Part model, mm, in its own coordinate system. A direction names the side the tool comes from. Round coordinates to 2 decimals unless told otherwise and drop trailing zeros. Loops run counter-clockwise (first coordinate to the right, second up) from the corner with the lowest first, then second, coordinate; pieces in that order, holes last.
(1) Mould opens along Z. For faces 4 (the face through (0, 0, 12.7)), 5 (the face through (-18, -12.785, 0)), 6 (the face through (1, 21.505, 11)) say: +Z half, -Z half, draft (parallel to the pull), parting line (faces both ways), or undercut.
(2) Tool access for faces 1 (the face through (23, -8.975, 41)), 2 (the face through (20, 0, -6.35)), 3 (the face through (-9.57, 5.85, 9.57)): list every direction of +Z, -Z, +X, -X, +Y, -Y with a clear straight run to the whole face (end or side of a thin tool).
(3) Flat gauge pins, fed straight in: pin 1 (5 mm diameter, centred on x = 8.5, y = 8, fed in from +Z); pin 2 (4 mm diameter, centred on x = 15.5, y = -12, fed in from -Z); pin 3 (8 mm diameter, centred on x = 6.5, z = -12.5, fed in from +Y); pin 4 (5 mm diameter, centred on x = 22, y = -1.5, fed in from +Z). Where does each tip first touch, or does it go through?
(4) Probe probe 1 along Y at (x, z) = (12.7, 10.25); probe 2 along X at (y, z) = (-11, -7) (3 decimals); probe 3 along X at (y, z) = (12, 33) (3 decimals). List the from-to ranges inside material, lowest first.
(5) Cut at B-B on z = 31.5. List the corners of the cut face in (x, y) (3 decimals), then the cut area to 3 significant figures.
(6) Cut at C-C on x = -16. List the corners of the cut face in (y, z).
Autodesk Inventor part; units mm, degrees
ref_plane "YZ Plane" through (0, 0, 0) normal (1, 0, 0) x (0, 1, 0)
ref_plane "XZ Plane" through (0, 0, 0) normal (0, 1, 0) x (-1, 0, 0)
ref_plane "XY Plane" through (0, 0, 0) normal (0, 0, 1) x (1, 0, 0)
sketch "Sketch1" plane through (0, 0, 0) normal (0, 0, 1) x (1, 0, 0)
  line L0 (-15.24, 10.0753) -> (16.51, 10.0753)
  line L1 (16.51, 10.0753) -> (16.51, -15.3247)
  line L2 (16.51, -15.3247) -> (-15.24, -15.3247)
  line L3 (-15.24, -15.3247) -> (-15.24, 10.0753)
  circle A0 centre (-11.43, 6.2653) radius 1.905
  circle A1 centre (-11.43, -6.4347) radius 1.905
  circle A2 centre (12.7, 6.2653) radius 1.905
  circle A3 centre (12.7, -6.4347) radius 1.905
  point P0 (0, 0)
  dimension "d0" = 31.75
  dimension "d1" = 25.4
  dimension "d10" = 3.81
  dimension "d11" = 8.89
  dimension "d12" = 3.81
  dimension "d13" = 3.81
  dimension "d14" = 8.89
  dimension "d15" = 3.81
  dimension "d16" = 3.81
  dimension "d17" = 3.81
  dimension "d18" = 3.81
  dimension "d19" = 3.81
  dimension "d20" = 3.81
  dimension "d21" = 3.81
  dimension "d22" = 8.89
extrude "Extrusion1" add sketch "Sketch1" along normal blind 6.35
sketch "Sketch2" plane through (0, 0, 6.35) normal (0, 0, 1) x (1, 0, 0)
  line L0 (-24.765, 16.4253) -> (26.035, 16.4253)
  line L1 (26.035, 16.4253) -> (26.035, -21.6747)
  line L2 (26.035, -21.6747) -> (-24.765, -21.6747)
  line L3 (-24.765, -21.6747) -> (-24.765, 16.4253)
  line L4 (16.51, -15.3247) -> (16.51, 10.0753)
  line L5 (-15.24, 10.0753) -> (-15.24, -15.3247)
  line L6 (16.51, 10.0753) -> (-15.24, 10.0753)
  point P0 (0, 0)
  dimension "d25" = 50.8
  dimension "d26" = 38.1
  dimension "d27" = 9.525
  dimension "d29" = 9.525
  dimension "d30" = 6.35
extrude "Extrusion2" add sketch "Sketch2" along normal blind 6.35
sketch "Sketch3" plane through (0, 0, 6.35) normal (0, 0, -1) x (-1, 0, 0)
  line L0 (24.765, -21.6747) -> (24.765, 16.4253)
  circle A0 centre (11.43, 6.2653) radius 1.905
  line L1 (24.765, 16.4253) -> (-26.035, 16.4253)
  circle A1 centre (11.43, -6.4347) radius 1.905
  line L2 (-26.035, -21.6747) -> (24.765, -21.6747)
  line L3 (-26.035, 16.4253) -> (-26.035, -21.6747)
  point P0 (0, 0)
  point P1 (-12.7, -6.4347)
  point P2 (-12.7, 6.2653)
  dimension "d33" = 13.335
  dimension "d34" = 10.16
  dimension "d35" = 13.335
  dimension "d36" = 15.24
  dimension "d37" = 13.335
  dimension "d38" = 10.16
  dimension "d39" = 15.24
  dimension "d40" = 13.335
hole "Hole1" at (-11.43, 6.2653, 6.35) at (-11.43, -6.4347, 6.35) at (12.7, -6.4347, 6.35) at (12.7, 6.2653, 6.35) direction (0, 0, 1) diameter 3.81 end through all
sketch "Sketch4" plane through (0, 0, 12.7) normal (0, 0, 1) x (1, 0, 0)
  line L0 (26.035, 16.4253) -> (26.035, -21.6747)
  line L1 (26.035, 16.4253) -> (19.685, 16.4253)
  line L2 (19.685, 16.4253) -> (19.685, -21.6747)
  line L3 (19.685, -21.6747) -> (26.035, -21.6747)
  line L4 (26.035, -21.6747) -> (26.035, 16.4253)
  line L5 (-24.765, 16.4253) -> (26.035, 16.4253)
  line L6 (-24.765, 16.4253) -> (-18.415, 16.4253)
  line L7 (-18.415, 16.4253) -> (-18.415, -21.6747)
  line L8 (-18.415, -21.6747) -> (-24.765, -21.6747)
  line L9 (-24.765, -21.6747) -> (-24.765, 16.4253)
  point P0 (0, 0)
  dimension "d48" = 6.35
  dimension "d49" = 6.35
extrude "Extrusion3" add sketch "Sketch4" along normal blind 34.925
sketch "Sketch5" plane through (26.035, -21.6747, 6.35) normal (1, 0, 0) x (0, 0, -1)
  line L0 (-41.2903, 25.4) -> (-28.2305, 25.4)
  line L1 (-28.2305, 25.4) -> (-28.2305, 12.7)
  line L2 (-28.2305, 12.7) -> (-41.2903, 12.7)
  line L3 (-41.2903, 12.7) -> (-41.2903, 25.4)
  line L4 (0, 38.1) -> (-41.275, 38.1)
  point P0 (6.35, 21.6747)
  dimension "d52" = 12.7
  dimension "d53" = 12.7
extrude "Extrusion4" cut sketch "Sketch5" against normal through all
sketch "Sketch6" plane through (0, 0, 6.35) normal (0, 0, -1) x (-1, 0, 0)
  point P0 (0, 0)
sketch "Sketch7" plane through (0, 0, 6.35) normal (0, 0, -1) x (-1, 0, 0)
  line L0 (-26.035, 16.4253) -> (-26.035, -21.6747)
  line L1 (24.765, -21.6747) -> (18.415, -21.6747)
  line L2 (-26.035, 16.4253) -> (24.765, 16.4253)
  line L3 (24.765, 16.4253) -> (24.765, -21.6747)
  line L4 (24.765, -21.6747) -> (-26.035, -21.6747)
  line L5 (-26.035, -21.6747) -> (-26.035, 16.4253)
  point P0 (0, 0)
extrude "Extrusion5" add sketch "Sketch7" along normal blind 32.385
sketch "Sketch8" plane through (-18.415, -21.6747, 12.7) normal (0, -1, 0) x (1, 0, 0)
  line L0 (44.45, -38.735) -> (-6.35, -38.735)
  line L1 (44.45, 34.925) -> (44.45, -38.735)
  line L2 (0, 0) -> (38.1, 0)
  line L3 (-6.35, 34.925) -> (-6.35, -38.735)
  point P0 (18.415, -12.7)
  point P1 (19.05, -19.3675)
  dimension "d60" = 19.3675
  dimension "d61" = 25.4
  dimension "d62" = 19.3675
  dimension "d63" = 25.4
hole "Hole2" at (0.635, -21.6747, -6.6675) direction (0, 1, 0) diameter 26.797 end through all
fillet "Fillet3" radius 12.7 2 edges at (-24.765, -2.6247, -26.035) (26.035, -2.6247, -26.035)
sketch "Sketch9" plane through (0, 0, 12.7) normal (0, 0, 1) x (1, 0, 0)
  circle A0 centre (12.7, -6.4347) radius 1.905
  circle A1 centre (-11.43, -6.4347) radius 1.905
  circle A2 centre (-11.43, 6.2653) radius 1.905
  line L0 (-18.415, -21.6747) -> (19.685, -21.6747)
  line L1 (26.035, 3.7253) -> (26.035, -8.9747)
  circle A3 centre (12.7, 6.2653) radius 1.905
  circle A4 centre (-11.43, -6.4347) radius 1.905
  circle A5 centre (12.7, 6.2653) radius 1.905
  line L2 (19.685, 16.4253) -> (-18.415, 16.4253)
  point P0 (0, 0)
  dimension "d73" = 15.24
  dimension "d74" = 13.335
  dimension "d75" = 12.7
  dimension "d76" = 24.13
  dimension "d77" = 24.13
  dimension "d78" = 3.81
  dimension "d79" = 3.81
  dimension "d80" = 12.7
  dimension "d81" = 3.81
  dimension "d82" = 10.16
  dimension "d83" = 24.13
extrude "Extrusion6" cut sketch "Sketch9" against normal blind 19.05
sketch "Sketch10" plane through (26.035, 3.7253, 47.625) normal (1, 0, 0) x (0, 0, -1)
  line L0 (41.275, 8.89) -> (53.975, 8.89)
  line L1 (53.975, 8.89) -> (53.975, -16.51)
  line L2 (53.975, -16.51) -> (41.275, -16.51)
  line L3 (41.275, -16.51) -> (41.275, 8.89)
  line L4 (34.925, -25.4) -> (34.925, 12.7)
  line L5 (0, 12.7) -> (60.96, 12.7)
  point P0 (47.625, -3.7253)
  dimension "d86" = 12.7
  dimension "d87" = 25.4
  dimension "d88" = 6.35
  dimension "d91" = 3.81
extrude "Extrusion7" cut sketch "Sketch10" against normal through all
thicken "Thicken1" operation add thickness 5.08 both sides no extend neighbours yes toward (0, 1, 0) faces at (-22.6483, 16.4253, 15.6633)
sketch "Sketch11" plane through (-18.415, 21.5053, 12.7) normal (0, 1, 0) x (1, 0, 0)
  point P0 (18.415, 12.7)
sketch "Sketch12" plane through (-24.765, -21.6747, 47.625) normal (-1, 0, 0) x (0, 0, 1)
  line L0 (-60.96, 43.18) -> (0, 43.18)
  line L1 (0, 0) -> (-60.96, 0)
  point P0 (-47.625, 21.6747)
sketch "Sketch13" plane through (-18.415, 21.5053, 12.7) normal (0, 1, 0) x (1, 0, 0)
  line L0 (44.45, -34.925) -> (44.45, 26.035)
  line L1 (-6.35, 26.035) -> (-6.35, -34.925)
  point P0 (18.415, 12.7)
  dimension "d95" = 50.8
equation "\"d12\" = d13"
equation "\"d15\" = d10"
equation "\"d16\" = d10"
equation "\"d17\" = d10"
equation "\"d19\" = d13"
equation "\"d20\" = d13"
equation "\"d21\" = d20"
equation "\"d22\" = d14"
equation "\"d77\" = d76"
equation "\"d79\" = d78"
properties part number "Vertical Seeder Rod spacer"
Final values:
1. face 4: +Z half
1. face 5: undercut
1. face 6: draft
2. face 1: +Z, +X, -X
2. face 2: +X, -X
2. face 3: +Z
3. pin 1: stops at z = 12.7
3. pin 2: stops at z = -26.03
3. pin 3: passes through
3. pin 4: stops at z = 34.58
4. probe 1: y = -21.67 to -8.34, -4.53 to 4.36, 8.17 to 21.51
4. probe 2: x = -24.765 to -12.759, 14.029 to 26.035
4. probe 3: x = -24.765 to -18.415, 19.685 to 26.035
5. outline: (-24.765, -21.675) - (-18.415, -21.675) - (-18.415, 21.505) - (-24.765, 21.505) - close; (19.685, -21.675) - (26.035, -21.675) - (26.035, 21.505) - (19.685, 21.505) - close
5. area: 548 mm2
6. outline: (-21.67, -25.41) - (21.51, -25.41) - (21.51, 12.7) - (-21.67, 12.7) - close; hole (-12.78, -6.35) - (12.62, -6.35) - (12.62, 6.35) - (-12.78, 6.35) - close
